For this review, take the finished solid that the model builds, in its own axes (mm). A direction names the side the tool comes from. Give positions to 0.01 mm unless a question says otherwise; leave off trailing zeros. Order: outer loops, then holes, each group sorted by start corner. A loop starts at its lowest first (then second) coordinate and runs counter-clockwise, first axis right, second up. Notation, with made-up numbers: (-14, -29.5) -> (20, -29.5) arc R25 ccw to (20, -8.5) -> close; hole circle Ø10 at (12, 46). An arc over 180 degrees is marked (long way). Return JSON: item names as keys, results as strings. Group by question number.
1) Add section A-A (y = 75). Give the boundary of the cut face in (x, z).
2) Add section D-D (y = 48). Give the boundary of the cut face in (x, z), then the cut area to 3 significant figures.
3) The part is to be moulded in two halves that separate along Y. For faces 3 (the face through (195, 89, 6)), 4 (the face through (195, 57, 8)), 5 (the face through (154.22, 76.8, 5.97)), 6 (the face through (160.18, 75, 6)), say which applies: released by +Y, released by -Y, zero draft, split by the parting line, or undercut.
4) Add section B-B (z = 7.25). Give the boundary of the cut face in (x, y), then the cut area to 3 significant figures.
5) To check wall thickness, follow line 1 along X through (y, z) = (86.5, 4.5); line 2 along Y through (x, z) = (205, 6.1); line 3 along Y through (x, z) = (186.5, 7). State the ranges of each line that lie inside material, in increasing order.
6) For faces 1 (the face through (229.039, 83.797, 5.972)), 2 (the face through (195, 57, 4)), list the 3-axis set-ups (+Z, -Z, +X, -X, +Y, -Y) from which the entire face can be reached by the end or side of a thin tool; tool diameter is ignored.
7) Add section C-C (x = 180). Give the boundary of the cut face in (y, z).
8) Insertion check: P1, Ø1.2, axis at y = 74, z = 5.5, coming from the -X side; P2, Ø1, axis at y = 62.5, z = 7, coming from the -X side (3 decimals); P3, Ø2, axis at x = 204.5, z = 7, coming from the +Y side. Each pin has a flat end and moves straight along its axis. Give the tip position at first contact, or say it passes through.
from build123d import *

# Parameters (mm, degrees)
SKETCH_R        = 41
PAD_DEPTH       = 4
SKETCH004_W     = 40
SKETCH004_H     = 4
POCKET002_DEPTH = 8.001


with BuildPart() as part:
    # Sketch → Pad (new body)
    with BuildSketch(Plane.XY.offset(4)):
        with Locations((195.179598, 75)):
            Circle(SKETCH_R)
        with BuildLine():
            Line((195.179598, 65), (226.179598, 65))
            ThreePointArc((226.179598, 65), (229.008025, 66.171573), (230.179598, 69))
            Line((230.179598, 69), (230.179598, 81))
            ThreePointArc((230.179598, 81), (229.008025, 83.828427), (226.179598, 85))
            Line((226.179598, 85), (195.179598, 85))
            Line((195.179598, 85), (164.179598, 85))
            ThreePointArc((164.179598, 85), (161.351171, 83.828427), (160.179598, 81))
            Line((160.179598, 81), (160.179598, 69))
            ThreePointArc((160.179598, 69), (161.351171, 66.171573), (164.179598, 65))
            Line((164.179598, 65), (195.179598, 65))
        make_face(mode=Mode.SUBTRACT)
    extrude(amount=PAD_DEPTH)

    # Sketch004 → Pocket002 (cut, through all)
    with BuildSketch(Plane.XY):
        with Locations((195.179598, 63)):
            Rectangle(SKETCH004_W, SKETCH004_H)
        with Locations((195.179598, 87)):
            Rectangle(SKETCH004_W, SKETCH004_H)
    extrude(amount=POCKET002_DEPTH, mode=Mode.SUBTRACT)


solid = part.part
Evaluation:
{
 "1": {"outline": "(154.18, 4) -> (160.18, 4) -> (160.18, 8) -> (154.18, 8) -> close; (230.18, 4) -> (236.18, 4) -> (236.18, 8) -> (230.18, 8) -> close"},
 "2": {"outline": "(164.33, 4) -> (226.03, 4) -> (226.03, 8) -> (164.33, 8) -> close", "area": "247 mm^2"},
 "3": {"face 3": "undercut", "face 4": "zero draft", "face 5": "split by the parting line", "face 6": "undercut"},
 "4": {"outline": "circle Ø82 at (195.18, 75); hole (160.18, 69) arc R4 ccw to (164.18, 65) -> (175.18, 65) -> (175.18, 61) -> (215.18, 61) -> (215.18, 65) -> (226.18, 65) arc R4 ccw to (230.18, 69) -> (230.18, 81) arc R4 ccw to (226.18, 85) -> (215.18, 85) -> (215.18, 89) -> (175.18, 89) -> (175.18, 85) -> (164.18, 85) arc R4 ccw to (160.18, 81) -> close", "area": "3,570 mm^2"},
 "5": {"line 1": "155.83 to 175.18, 215.18 to 234.53", "line 2": "35.19 to 61, 89 to 114.81", "line 3": "34.93 to 61, 89 to 115.07"},
 "6": {"face 1": "+Z, -Z", "face 2": "-Z, +X, -X, +Y, -Y"},
 "7": {"outline": "(36.91, 4) -> (61, 4) -> (61, 8) -> (36.91, 8) -> close; (89, 4) -> (113.09, 4) -> (113.09, 8) -> (89, 8) -> close"},
 "8": {"P1": "x = 154.18", "P2": "x = 155.975", "P3": "y = 115.15"}
}
